Geometry: final body of the model. Coordinates: model frame, mm. A direction names the side the tool comes from. Give positions to 0.01 mm unless a question says otherwise; leave off trailing zeros. Order: outer loops, then holes, each group sorted by start corner. A loop starts at its lowest first (then second) coordinate and runs counter-clockwise, first axis right, second up. Notation, with made-up numbers: (66.25, 78) -> (76.25, 78) arc R10 ccw to (76.25, 82) -> close; hole circle Ø9 at (75, 20). An arc over 180 degrees is marked (long way). One line per question, with ' | ' between items.
from build123d import *

# Parameters (mm, degrees)
SKETCH1_W               = 22
SKETCH1_H               = 52
BOSS_EXTRUDE1_DEPTH     = 7
SKETCH2_W               = 20.1
SKETCH2_H               = 50.1
CUT_EXTRUDE1_DEPTH      = 6
FILLET1_R               = 1
SKETCH4_W               = 1.5
SKETCH4_H               = 10
CUT_EXTRUDE3_DEPTH      = 8
SKETCH5_R               = 1.55
CUT_EXTRUDE4_DEPTH      = 0.2
SKETCH6_R               = 1.55
CUT_EXTRUDE5_DEPTH      = 0.2
SKETCH7_R               = 0.8
CUT_EXTRUDE6_DEPTH      = 7
CUT_EXTRUDE6_DEPTH_BACK = 2
CUT_EXTRUDE7_REACH      = 3
SKETCH8_R               = 0.8
CUT_EXTRUDE9_REACH      = 3
SKETCH9_R               = 0.8
CUT_EXTRUDE10_REACH     = 3
SKETCH10_R              = 0.8
CUT_EXTRUDE11_REACH     = 3
SKETCH11_R              = 0.8
CUT_EXTRUDE12_REACH     = 3
SKETCH12_R              = 0.8
CUT_EXTRUDE13_REACH     = 3
SKETCH13_R              = 0.8
CUT_EXTRUDE14_REACH     = 3
SKETCH14_R              = 0.8
CUT_EXTRUDE15_REACH     = 3
SKETCH15_R              = 0.8
CUT_EXTRUDE16_REACH     = 3
SKETCH16_R              = 0.8


with BuildPart() as part:
    # Sketch1 → Boss-Extrude1 (new body)
    with BuildSketch(Plane(origin=(0, 0, 0), x_dir=(1, 0, 0), z_dir=(0, 1, 0))):
        Rectangle(SKETCH1_W, SKETCH1_H)
    extrude(amount=BOSS_EXTRUDE1_DEPTH)

    # Sketch2 → Cut-Extrude1 (cut)
    with BuildSketch(Plane(origin=(0, 7, 0), x_dir=(1, 0, 0), z_dir=(0, 1, 0))):
        Rectangle(SKETCH2_W, SKETCH2_H)
    extrude(amount=-CUT_EXTRUDE1_DEPTH, mode=Mode.SUBTRACT)

    # Fillet1
    fillet1_edges = [part.edges().sort_by_distance(p)[0] for p in [
        (11, 3.5, 26),
        (-11, 3.5, 26),
        (-11, 3.5, -26),
        (11, 3.5, -26),
    ]]
    fillet(fillet1_edges, radius=FILLET1_R)

    # Sketch4 → Cut-Extrude3 (cut, through all)
    with BuildSketch(Plane.XZ):
        with Locations((-10.25, 0)):
            Rectangle(SKETCH4_W, SKETCH4_H)
        with Locations((10.25, 0)):
            Rectangle(SKETCH4_W, SKETCH4_H)
    extrude(amount=-CUT_EXTRUDE3_DEPTH, mode=Mode.SUBTRACT)

    # Sketch5 → Cut-Extrude4 (cut)
    with BuildSketch(Plane(origin=(0, 1, 0), x_dir=(1, 0, 0), z_dir=(0, 1, 0))):
        with Locations((0, -17.55)):
            Circle(SKETCH5_R)
    extrude(amount=-CUT_EXTRUDE4_DEPTH, mode=Mode.SUBTRACT)

    # Sketch6 → Cut-Extrude5 (cut)
    with BuildSketch(Plane(origin=(0, 1, 0), x_dir=(1, 0, 0), z_dir=(0, 1, 0))):
        with Locations((0, 17.05)):
            Circle(SKETCH6_R)
    extrude(amount=-CUT_EXTRUDE5_DEPTH, mode=Mode.SUBTRACT)

    # Sketch7 → Cut-Extrude6 (cut, two sides)
    with BuildSketch(Plane(origin=(0, 1, 0), x_dir=(1, 0, 0), z_dir=(0, 1, 0))) as cut_extrude6_sk:
        with Locations((-8.15, -23)):
            Circle(SKETCH7_R)
    extrude(amount=CUT_EXTRUDE6_DEPTH, mode=Mode.SUBTRACT)
    extrude(cut_extrude6_sk.sketch, amount=-CUT_EXTRUDE6_DEPTH_BACK, mode=Mode.SUBTRACT)

    # Sketch8 → Cut-Extrude7 (cut, up to next)
    with BuildSketch(Plane(origin=(0, 1, 0), x_dir=(1, 0, 0), z_dir=(0, 1, 0)), mode=Mode.PRIVATE) as cut_extrude7_sk1:
        with Locations((-5.75, -12.3)):
            Circle(SKETCH8_R)
    cut_extrude7_tool1 = extrude(cut_extrude7_sk1.sketch, amount=-CUT_EXTRUDE7_REACH, mode=Mode.PRIVATE) & part.part
    add(cut_extrude7_tool1.solids().sort_by_distance((-5.75, 1, 12.3))[0], mode=Mode.SUBTRACT)
    # Sketch8 → Cut-Extrude7 (cut, up to next)
    with BuildSketch(Plane(origin=(0, 1, 0), x_dir=(1, 0, 0), z_dir=(0, 1, 0)), mode=Mode.PRIVATE) as cut_extrude7_sk2:
        with Locations((5, -12.3)):
            Circle(SKETCH8_R)
    cut_extrude7_tool2 = extrude(cut_extrude7_sk2.sketch, amount=-CUT_EXTRUDE7_REACH, mode=Mode.PRIVATE) & part.part
    add(cut_extrude7_tool2.solids().sort_by_distance((5, 1, 12.3))[0], mode=Mode.SUBTRACT)

    # Sketch9 → Cut-Extrude9 (cut, up to next)
    with BuildSketch(Plane(origin=(0, 1, 0), x_dir=(1, 0, 0), z_dir=(0, 1, 0)), mode=Mode.PRIVATE) as cut_extrude9_sk1:
        with Locations((-5.75, -9.5)):
            Circle(SKETCH9_R)
    cut_extrude9_tool1 = extrude(cut_extrude9_sk1.sketch, amount=-CUT_EXTRUDE9_REACH, mode=Mode.PRIVATE) & part.part
    add(cut_extrude9_tool1.solids().sort_by_distance((-5.75, 1, 9.5))[0], mode=Mode.SUBTRACT)
    # Sketch9 → Cut-Extrude9 (cut, up to next)
    with BuildSketch(Plane(origin=(0, 1, 0), x_dir=(1, 0, 0), z_dir=(0, 1, 0)), mode=Mode.PRIVATE) as cut_extrude9_sk2:
        with Locations((5, -9.5)):
            Circle(SKETCH9_R)
    cut_extrude9_tool2 = extrude(cut_extrude9_sk2.sketch, amount=-CUT_EXTRUDE9_REACH, mode=Mode.PRIVATE) & part.part
    add(cut_extrude9_tool2.solids().sort_by_distance((5, 1, 9.5))[0], mode=Mode.SUBTRACT)

    # Sketch10 → Cut-Extrude10 (cut, up to next)
    with BuildSketch(Plane(origin=(0, 1, 0), x_dir=(1, 0, 0), z_dir=(0, 1, 0)), mode=Mode.PRIVATE) as cut_extrude10_sk1:
        with Locations((-5.75, -6.8)):
            Circle(SKETCH10_R)
    cut_extrude10_tool1 = extrude(cut_extrude10_sk1.sketch, amount=-CUT_EXTRUDE10_REACH, mode=Mode.PRIVATE) & part.part
    add(cut_extrude10_tool1.solids().sort_by_distance((-5.75, 1, 6.8))[0], mode=Mode.SUBTRACT)
    # Sketch10 → Cut-Extrude10 (cut, up to next)
    with BuildSketch(Plane(origin=(0, 1, 0), x_dir=(1, 0, 0), z_dir=(0, 1, 0)), mode=Mode.PRIVATE) as cut_extrude10_sk2:
        with Locations((5, -6.837159935)):
            Circle(SKETCH10_R)
    cut_extrude10_tool2 = extrude(cut_extrude10_sk2.sketch, amount=-CUT_EXTRUDE10_REACH, mode=Mode.PRIVATE) & part.part
    add(cut_extrude10_tool2.solids().sort_by_distance((5, 1, 6.83716))[0], mode=Mode.SUBTRACT)

    # Sketch11 → Cut-Extrude11 (cut, up to next)
    with BuildSketch(Plane(origin=(0, 1, 0), x_dir=(1, 0, 0), z_dir=(0, 1, 0)), mode=Mode.PRIVATE) as cut_extrude11_sk1:
        with Locations((-0.3, -12.3)):
            Circle(SKETCH11_R)
    cut_extrude11_tool1 = extrude(cut_extrude11_sk1.sketch, amount=-CUT_EXTRUDE11_REACH, mode=Mode.PRIVATE) & part.part
    add(cut_extrude11_tool1.solids().sort_by_distance((-0.3, 1, 12.3))[0], mode=Mode.SUBTRACT)

    # Sketch12 → Cut-Extrude12 (cut, up to next)
    with BuildSketch(Plane(origin=(0, 1, 0), x_dir=(1, 0, 0), z_dir=(0, 1, 0)), mode=Mode.PRIVATE) as cut_extrude12_sk1:
        with Locations((3.95, 12.05)):
            Circle(SKETCH12_R)
    cut_extrude12_tool1 = extrude(cut_extrude12_sk1.sketch, amount=-CUT_EXTRUDE12_REACH, mode=Mode.PRIVATE) & part.part
    add(cut_extrude12_tool1.solids().sort_by_distance((3.95, 1, -12.05))[0], mode=Mode.SUBTRACT)
    # Sketch12 → Cut-Extrude12 (cut, up to next)
    with BuildSketch(Plane(origin=(0, 1, 0), x_dir=(1, 0, 0), z_dir=(0, 1, 0)), mode=Mode.PRIVATE) as cut_extrude12_sk2:
        with Locations((-6.8, 12.05)):
            Circle(SKETCH12_R)
    cut_extrude12_tool2 = extrude(cut_extrude12_sk2.sketch, amount=-CUT_EXTRUDE12_REACH, mode=Mode.PRIVATE) & part.part
    add(cut_extrude12_tool2.solids().sort_by_distance((-6.8, 1, -12.05))[0], mode=Mode.SUBTRACT)

    # Sketch13 → Cut-Extrude13 (cut, up to next)
    with BuildSketch(Plane(origin=(0, 1, 0), x_dir=(1, 0, 0), z_dir=(0, 1, 0)), mode=Mode.PRIVATE) as cut_extrude13_sk1:
        with Locations((3.95, 9.3)):
            Circle(SKETCH13_R)
    cut_extrude13_tool1 = extrude(cut_extrude13_sk1.sketch, amount=-CUT_EXTRUDE13_REACH, mode=Mode.PRIVATE) & part.part
    add(cut_extrude13_tool1.solids().sort_by_distance((3.95, 1, -9.3))[0], mode=Mode.SUBTRACT)
    # Sketch13 → Cut-Extrude13 (cut, up to next)
    with BuildSketch(Plane(origin=(0, 1, 0), x_dir=(1, 0, 0), z_dir=(0, 1, 0)), mode=Mode.PRIVATE) as cut_extrude13_sk2:
        with Locations((-6.8, 9.3)):
            Circle(SKETCH13_R)
    cut_extrude13_tool2 = extrude(cut_extrude13_sk2.sketch, amount=-CUT_EXTRUDE13_REACH, mode=Mode.PRIVATE) & part.part
    add(cut_extrude13_tool2.solids().sort_by_distance((-6.8, 1, -9.3))[0], mode=Mode.SUBTRACT)

    # Sketch14 → Cut-Extrude14 (cut, up to next)
    with BuildSketch(Plane(origin=(0, 1, 0), x_dir=(1, 0, 0), z_dir=(0, 1, 0)), mode=Mode.PRIVATE) as cut_extrude14_sk1:
        with Locations((3.9, 6.6)):
            Circle(SKETCH14_R)
    cut_extrude14_tool1 = extrude(cut_extrude14_sk1.sketch, amount=-CUT_EXTRUDE14_REACH, mode=Mode.PRIVATE) & part.part
    add(cut_extrude14_tool1.solids().sort_by_distance((3.9, 1, -6.6))[0], mode=Mode.SUBTRACT)
    # Sketch14 → Cut-Extrude14 (cut, up to next)
    with BuildSketch(Plane(origin=(0, 1, 0), x_dir=(1, 0, 0), z_dir=(0, 1, 0)), mode=Mode.PRIVATE) as cut_extrude14_sk2:
        with Locations((-6.85, 6.6)):
            Circle(SKETCH14_R)
    cut_extrude14_tool2 = extrude(cut_extrude14_sk2.sketch, amount=-CUT_EXTRUDE14_REACH, mode=Mode.PRIVATE) & part.part
    add(cut_extrude14_tool2.solids().sort_by_distance((-6.85, 1, -6.6))[0], mode=Mode.SUBTRACT)

    # Sketch15 → Cut-Extrude15 (cut, up to next)
    with BuildSketch(Plane(origin=(0, 1, 0), x_dir=(1, 0, 0), z_dir=(0, 1, 0)), mode=Mode.PRIVATE) as cut_extrude15_sk1:
        with Locations((-1.6, 11.05)):
            Circle(SKETCH15_R)
    cut_extrude15_tool1 = extrude(cut_extrude15_sk1.sketch, amount=-CUT_EXTRUDE15_REACH, mode=Mode.PRIVATE) & part.part
    add(cut_extrude15_tool1.solids().sort_by_distance((-1.6, 1, -11.05))[0], mode=Mode.SUBTRACT)

    # Sketch16 → Cut-Extrude16 (cut, up to next)
    with BuildSketch(Plane(origin=(0, 1, 0), x_dir=(1, 0, 0), z_dir=(0, 1, 0)), mode=Mode.PRIVATE) as cut_extrude16_sk1:
        with Locations((-8.25, 17.05)):
            Circle(SKETCH16_R)
    cut_extrude16_tool1 = extrude(cut_extrude16_sk1.sketch, amount=-CUT_EXTRUDE16_REACH, mode=Mode.PRIVATE) & part.part
    add(cut_extrude16_tool1.solids().sort_by_distance((-8.25, 1, -17.05))[0], mode=Mode.SUBTRACT)


solid = part.part
1) Set-up query: faces 1 (the flat face through (10.05, 4, 15)), 2 (the flat face through (10.4, 3.5, 5)), 3 (the cylindrical face through (-6.37, 0.507, -12.725)). Return all of +Z, -Z, +X, -X, +Y, -Y with unobstructed straight access to the full face (end or side cutting, diameter ignored); none if empty.
Check result:
face 1: +Y | face 2: +X, +Y, -Y | face 3: +Y, -Y
2) Section D-D on x = 0. Return loops of the section in (y, z), plus the area to 3 significant figures.
Check result:
outline: (0, -26) -> (7, -26) -> (7, -25.05) -> (1, -25.05) -> (1, -18.6) -> (0.8, -18.6) -> (0.8, -15.5) -> (1, -15.5) -> (1, 11.56) -> (0, 11.56) -> close; (0, 13.04) -> (1, 13.04) -> (1, 16) -> (0.8, 16) -> (0.8, 19.1) -> (1, 19.1) -> (1, 25.05) -> (7, 25.05) -> (7, 26) -> (0, 26) -> close | area: 60.7 mm^2
3) Contact query for flat-ended pins moving along their axis: pin 1 Ø1.5 at (x, z) = (-7.5, 8.5) entering from +Y; pin 2 Ø0.8 at (x, y) = (-10.5, 4.5) entering from +Z (3 decimals). Output: stop coordinate, or through.
Check result:
pin 1: stops at y = 1 | pin 2: stops at z = 25.995
4) Section C-C on y = 5. Return loops of the section in (x, z).
Check result:
outline: (-11, -25) arc R1 ccw to (-10, -26) -> (10, -26) arc R1 ccw to (11, -25) -> (11, -5) -> (10.05, -5) -> (10.05, -25.05) -> (-10.05, -25.05) -> (-10.05, -5) -> (-11, -5) -> close; (-11, 5) -> (-10.05, 5) -> (-10.05, 25.05) -> (10.05, 25.05) -> (10.05, 5) -> (11, 5) -> (11, 25) arc R1 ccw to (10, 26) -> (-10, 26) arc R1 ccw to (-11, 25) -> close
5) Section B-B on z = 23. Return loops of the section in (x, y).
Check result:
outline: (-11, 0) -> (-8.95, 0) -> (-8.95, 1) -> (-10.05, 1) -> (-10.05, 7) -> (-11, 7) -> close; (-7.35, 0) -> (11, 0) -> (11, 7) -> (10.05, 7) -> (10.05, 1) -> (-7.35, 1) -> close
6) Material intervals for probe 1 along X at (y, z) = (0.5, -9.3); probe 2 along X at (y, z) = (0.3, 9.5); probe 3 along Z at (x, y) = (5, 0.2), sorted ascending. Write a range as from..to.
Check result:
probe 1: x = -11..-7.6, -6..3.15, 4.75..11 | probe 2: x = -11..-6.55, -4.95..4.2, 5.8..11 | probe 3: z = -26..6.04, 7.64..8.7, 10.3..11.5, 13.1..26
7) Section A-A on z = 12.3. Return loops of the section in (x, y).
Check result:
outline: (-11, 0) -> (-6.55, 0) -> (-6.55, 1) -> (-10.05, 1) -> (-10.05, 7) -> (-11, 7) -> close; (-4.95, 0) -> (-1.1, 0) -> (-1.1, 1) -> (-4.95, 1) -> close; (0.5, 0) -> (4.2, 0) -> (4.2, 1) -> (0.5, 1) -> close; (5.8, 0) -> (11, 0) -> (11, 7) -> (10.05, 7) -> (10.05, 1) -> (5.8, 1) -> close
8) Pull-direction query (Z, two-part tool) for faces 4 (the flat face through (0, 0, 0)), 5 (the flat face through (0, 3, -26)), 6 (the cylindrical face through (-5.854, 0.507, 8.707)); classes: +Z half, -Z half, draft (parallel to the pull), parting line (faces both ways), or undercut.
Check result:
face 4: draft | face 5: -Z half | face 6: undercut
